Answer from the drawing. Dimensions are ordinates in mm from the lowest x, y and z of the part. Coordinates: 2 decimals unless noted, no trailing zeros. Write each loop counter-clockwise with the first axis right and the second up, starting at its lowest first coordinate (ties: lowest second). Pieces come first, ordered by that corner, then holes.
(1) The part is cut by section D-D, the plane x = 563. Determine the outline of the cut face in (y, z), and give its area (3 significant figures).
(2) The part is cut by section C-C, the plane z = 8.5. State how many separate pieces and enclosed holes the cut face has, and give its area (3 significant figures).
(3) Given pin 1 (7.5 mm diameter, centred on y = 21.5, z = 17.5, fed in from +X), flat-ended and moving along its own axis, determine where the tip first touches the part or whether it passes through.
(4) Straight lines are drawn through the part: line 1 along Y through (x, z) = (342.9, 11.25) (3 decimals); line 2 along X through (y, z) = (219.5, 3); line 3 along X through (y, z) = (42.5, 14.5) (1 decimal). For each, find the intervals that lie inside material, in ascending order.
(5) The part is cut by section B-B, the plane x = 342.9. Determine the outline of the cut face in (y, z) (3 decimals), and give its area (3 significant figures).
(6) The part is cut by section A-A, the plane y = 317.5. Determine the outline of the cut face in (x, z) (3 decimals).
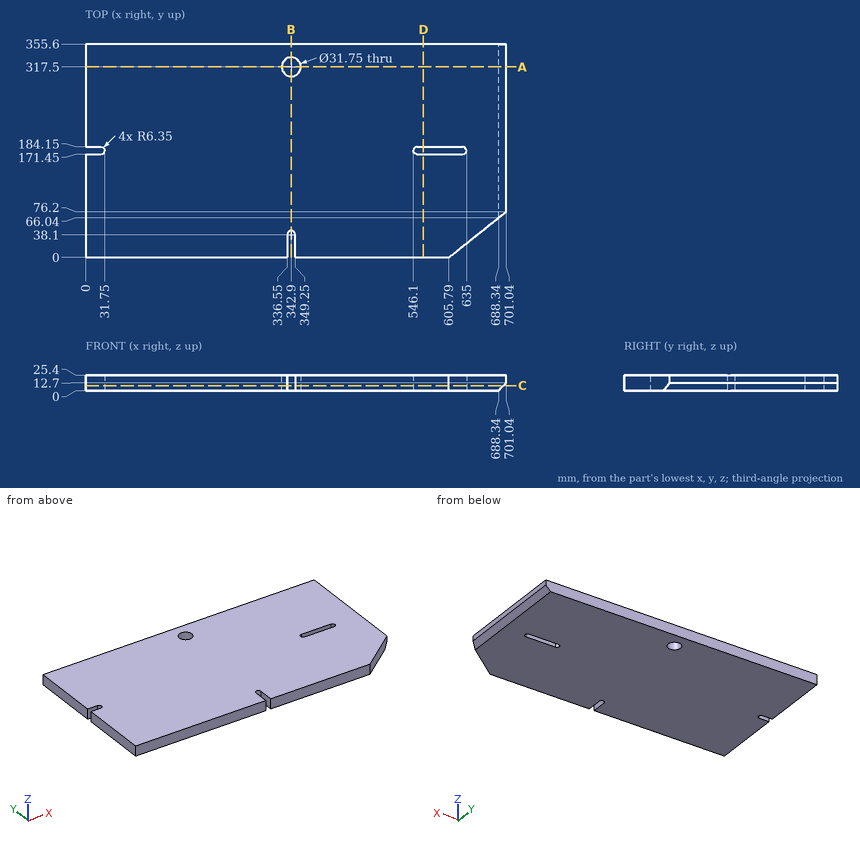
Computed:
1. outline: (0, 0) - (171.45, 0) - (171.45, 25.4) - (0, 25.4) - close; (184.15, 0) - (355.6, 0) - (355.6, 25.4) - (184.15, 25.4) - close
1. area: 8,710 mm2
2. separate pieces: 1
2. enclosed holes: 2
2. area: 242,000 mm2
3. pin 1: stops at x = 637.35
4. line 1: y = 44.45 to 301.625, 333.375 to 355.6
4. line 2: x = 0 to 691.34
4. line 3: x = 0 to 338.3, 347.5 to 658.9
5. outline: (44.45, 0) - (301.625, 0) - (301.625, 25.4) - (44.45, 25.4) - close; (333.375, 0) - (355.6, 0) - (355.6, 25.4) - (333.375, 25.4) - close
5. area: 7,100 mm2
6. outline: (0, 0) - (327.025, 0) - (327.025, 25.4) - (0, 25.4) - close; (358.775, 0) - (688.34, 0) - (701.04, 12.7) - (701.04, 25.4) - (358.775, 25.4) - close
